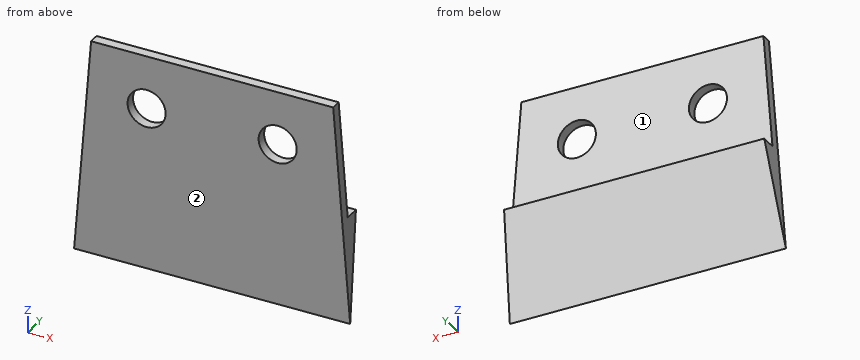
```python
from build123d import *

# Parameters (mm, degrees)
SKETCH1_R                       = 2.8448
BOSS_EXTRUDE1_DEPTH             = 1.524
BOSS_EXTRUDE2_REACH             = 31.04
BOSS_EXTRUDE2_DIRECTION_2_REACH = 31.04
CUT_EXTRUDE1_REACH              = 31.249
CUT_EXTRUDE1_DIRECTION_2_REACH  = 31.249


with BuildPart() as part:
    # Sketch1 → Boss-Extrude1 (new body)
    with BuildSketch(Plane(origin=(0, 0, 0), x_dir=(1, 0, 0), z_dir=(0, 1, 0))):
        Polygon((-20.228169231, 12.048978462), (21.021430769, 12.048978462), (18.481430769, -20.386821538), (-17.688169231, -20.386821538), align=None)
        with Locations(Location((-9.395069231, -12.411221538, 0), (0, 0, 90))):
            Circle(SKETCH1_R, mode=Mode.SUBTRACT)
        with Locations(Location((10.188330769, -12.411221538, 0), (0, 0, 90))):
            Circle(SKETCH1_R, mode=Mode.SUBTRACT)
    extrude(amount=BOSS_EXTRUDE1_DEPTH)

    # Boss-Extrude2: up to this plane
    boss_extrude2_end = Plane(origin=(19.95552113, 1.524, 1.562687637), z_dir=(-0.9969479165233839, 0, -0.07806953144270824))
    # Sketch4 → Boss-Extrude2 (add, up to the surface)
    with BuildSketch(Plane(origin=(0.396630769, 0, 0), x_dir=(0, 0, -1), z_dir=(1, 0, 0)), mode=Mode.PRIVATE) as boss_extrude2_sk1:
        Polygon((-3.114821538, 3.81), (-3.114821538, 1.524), (5.983458462, 1.524), align=None)
    boss_extrude2_tool1 = split(extrude(boss_extrude2_sk1.sketch, amount=BOSS_EXTRUDE2_REACH, mode=Mode.PRIVATE), bisect_by=boss_extrude2_end, keep=Keep.BOTH, mode=Mode.PRIVATE)
    add(boss_extrude2_tool1.solids().sort_by_distance((0.396631, 2.286, 0.082062))[0])

    # Boss-Extrude2 direction 2: up to this plane
    boss_extrude2_direction_2_end = Plane(origin=(-19.167094403, 1.524, 1.500947095), z_dir=(-0.9969479165233839, 0, 0.07806953144270846))
    # Sketch4 → Boss-Extrude2 direction 2 (add, up to the surface)
    with BuildSketch(Plane(origin=(0.396630769, 0, 0), x_dir=(0, 0, -1), z_dir=(1, 0, 0)), mode=Mode.PRIVATE) as boss_extrude2_direction_2_sk1:
        Polygon((-3.114821538, 3.81), (-3.114821538, 1.524), (5.983458462, 1.524), align=None)
    boss_extrude2_direction_2_tool1 = split(extrude(boss_extrude2_direction_2_sk1.sketch, amount=-BOSS_EXTRUDE2_DIRECTION_2_REACH, mode=Mode.PRIVATE), bisect_by=boss_extrude2_direction_2_end, keep=Keep.BOTH, mode=Mode.PRIVATE)
    add(boss_extrude2_direction_2_tool1.solids().sort_by_distance((0.396631, 2.286, 0.082062))[0])

    # Cut-Extrude1: up to this face of the body (flat: up to its plane)
    cut_extrude1_end = Plane(part.part.faces().sort_by_distance((-19.01379481, 1.026887005, 3.458582885))[0])
    # Sketch4<3> → Cut-Extrude1 (cut, up to the picked face)
    with BuildSketch(Plane(origin=(0.396630769, 0, 0), x_dir=(0, 0, -1), z_dir=(1, 0, 0)), mode=Mode.PRIVATE) as cut_extrude1_sk1:
        Polygon((12.048978462, 1.524), (5.983458462, 1.524), (12.048978462, 0), align=None)
    cut_extrude1_tool1 = split(extrude(cut_extrude1_sk1.sketch, amount=-CUT_EXTRUDE1_REACH, mode=Mode.PRIVATE), bisect_by=cut_extrude1_end, keep=Keep.BOTH, mode=Mode.PRIVATE)
    add(cut_extrude1_tool1.solids().sort_by(Axis((0.396631, 1.016, -10.027138), (-1, 0, 0)))[0], mode=Mode.SUBTRACT)

    # Cut-Extrude1 direction 2: up to this face of the body (flat: up to its plane)
    cut_extrude1_direction_2_end = Plane(part.part.faces().sort_by_distance((19.807056349, 1.026887005, 3.458582885))[0])
    # Sketch4<3> → Cut-Extrude1 direction 2 (cut, up to the picked face)
    with BuildSketch(Plane(origin=(0.396630769, 0, 0), x_dir=(0, 0, -1), z_dir=(1, 0, 0)), mode=Mode.PRIVATE) as cut_extrude1_direction_2_sk1:
        Polygon((12.048978462, 1.524), (5.983458462, 1.524), (12.048978462, 0), align=None)
    cut_extrude1_direction_2_tool1 = split(extrude(cut_extrude1_direction_2_sk1.sketch, amount=CUT_EXTRUDE1_DIRECTION_2_REACH, mode=Mode.PRIVATE), bisect_by=cut_extrude1_direction_2_end, keep=Keep.BOTH, mode=Mode.PRIVATE)
    add(cut_extrude1_direction_2_tool1.solids().sort_by(Axis((0.396631, 1.016, -10.027138), (1, 0, 0)))[0], mode=Mode.SUBTRACT)


solid = part.part
```
Geometry check sheet. Reference: the model listing, model coordinates, mm. Face numbers are marked on the shaded views. A direction names the side the tool comes from. Give positions to 0.01 mm unless a question says otherwise; leave off trailing zeros. Loops run counter-clockwise (first coordinate to the right, second up) from the corner with the lowest first, then second, coordinate; pieces in that order, holes last. Notation, with made-up numbers: M 76.5,66.5 L 125.5,66.5 A33 ccw 125.5,99.5 Z; hole C -3,73 d7. An arc over 180 degrees is marked long. Write item = value, one per line. Start each with the question number.
1. Section check B-B, the plane x = 12.5. Enter the section's corners in (y, z), plus the area to 3 significant figures.
2. Thickness scan on probe 1 along Y at (x, z) = (-3, 5); probe 2 along X at (y, z) = (2.8, 3); probe 3 along X at (y, z) = (0.4, 1). Record the ranges inside material, lowest first.
3. Tool access check on the marked faces 1 and 2. Record the directions out of +Z, -Z, +X, -X, +Y, -Y that give a thin tool (end or side, any length) a straight path to the whole face; none if there is none.
4. Section check C-C, the plane y = 1. Enter the section's corners in (x, z), plus the area to 3 significant figures.
5. Section check D-D, the plane x = 2. Enter the section's corners in (y, z), plus the area to 3 significant figures.
6. Go/stop test with flat-tipped pins: P1, Ø1.8, axis at x = -2, y = 2.5, coming from the +Z side; P2, Ø5, axis at x = -6.5, z = 8, coming from the +Y side; P3, Ø1.5, axis at x = -1, y = 2, coming from the +Z side; P4, Ø8, axis at x = 5, z = 2.5, coming from the +Y side. Record where each tip stops, or that it passes through.
7. Section check A-A, the plane z = 11. Enter the section's corners in (x, y), plus the area to 3 significant figures.
Values follow:
q1.outline = M 0,-12.05 L 3.81,3.11 L 1.52,3.11 L 1.52,10.75 L 0,10.75 Z; M 0,14.07 L 1.52,14.07 L 1.52,20.39 L 0,20.39 Z
q1.area = 50.2 mm^2
q2.probe_1 = 0 to 1.52
q2.probe_2 = -19.05 to 19.84
q2.probe_3 = -19.21 to 20
q3.face_1 = +Z, +X, -X, +Y
q3.face_2 = +Z, -Z, +X, -X, -Y
q4.outline = M -19.92,-8.07 L 20.71,-8.07 L 18.48,20.39 L -17.69,20.39 Z; hole C -9.4,12.41 d5.69; hole C 10.19,12.41 d5.69
q4.area = 1,040 mm^2
q5.outline = M 0,-12.05 L 3.81,3.11 L 1.52,3.11 L 1.52,20.39 L 0,20.39 Z
q5.area = 55.2 mm^2
q6.P1 = 3.11
q6.P2 = 1.52
q6.P3 = 20.39
q6.P4 = 3.81
q7.outline = M -18.42,0 L -11.87,0 L -11.87,1.52 L -18.42,1.52 Z; M -6.92,0 L 7.72,0 L 7.72,1.52 L -6.92,1.52 Z; M 12.66,0 L 19.22,0 L 19.22,1.52 L 12.66,1.52 Z
q7.area = 42.3 mm^2
